from build123d import *

# Parameters (mm, degrees)
SKETCH1_R                = 30
BOSS_EXTRUDE1_DEPTH      = 150
SKETCH3_R                = 57.769734486
BOSS_EXTRUDE2_DEPTH      = 25
BOSS_EXTRUDE2_DEPTH_BACK = 78


with BuildPart() as part:
    # Sketch1 → Boss-Extrude1 (new body)
    with BuildSketch(Plane(origin=(0, 0, 0), x_dir=(1, 0, 0), z_dir=(0, 1, 0))):
        Circle(SKETCH1_R)
    extrude(amount=BOSS_EXTRUDE1_DEPTH)

    # Sketch3 → Boss-Extrude2 (add, two sides)
    with BuildSketch(Plane(origin=(30, 0, 0), x_dir=(0, 0, -1), z_dir=(1, 0, 0))) as boss_extrude2_sk:
        with Locations((22.49423093, 77.731577971)):
            Circle(SKETCH3_R)
    extrude(amount=BOSS_EXTRUDE2_DEPTH)
    extrude(boss_extrude2_sk.sketch, amount=-BOSS_EXTRUDE2_DEPTH_BACK)


solid = part.part
Verification items for the finished model (mm, model axes). A direction names the side the tool comes from. Coordinates: 2 decimals unless noted, no trailing zeros. Order: outer loops, then holes, each group sorted by start corner. A loop starts at its lowest first (then second) coordinate and runs counter-clockwise, first axis right, second up. Notation, with made-up numbers: M 14,26.5 L 36,26.5 A30 ccw 36,57.5 Z; hole C 45,-7 d10. An arc over 180 degrees is marked long. One line per item, written item: value. Start each with the question number.
Item 1: Sectioned sample at B-B (x = 22.5). Enter the section's corners in (y, z).
Item 2: Scan lines: probe 1 along Y at (x, z) = (-24, -23.5); probe 2 along Y at (x, z) = (-43, -52); probe 3 along X at (y, z) = (13, 21.5). Record each from-to range of solid material in increasing order.
Item 3: Sectioned sample at D-D (z = -19). Enter the section's corners in (x, y), then the cut area to 3 significant figures.
Item 4: Sectioned sample at C-C (y = 125). Enter the section's corners in (x, z).
Item 5: Gauge pin test, flat ends, axial feed: pin 1 (1.5 mm diameter, centred on x = -27.5, y = 92, fed in from +Z); pin 2 (1.5 mm diameter, centred on x = -5.5, y = 114.5, fed in from -Z); pin 3 (1 mm diameter, centred on x = 18, z = -39.5, fed in from +Y). Record the tip position at first contact, or that the pin passes through.
Item 6: Sectioned sample at A-A (z = 0). Enter the section's corners in (x, y), then the cut area to 3 significant figures.
Item 7: Access from +Z, -Z, +X, -X, +Y, -Y to the whole of each face (thin tool, end or side, straight path). Record for faces 1 (the cylindrical face through (-6.503, 136.288, 29.287)), 2 (the cylindrical face through (-6.503, 14.517, 29.287)), 3 (the flat face through (0, 0, 0)).
Conclusion:
1. outline: M 0,-19.84 L 20.02,-19.84 A57.77 ccw long 135.44,-19.84 L 150,-19.84 L 150,19.84 L 117.04,19.84 A57.77 ccw 38.43,19.84 L 0,19.84 Z
2. probe 1: y = 19.97 to 135.49
2. probe 2: y = 28.07 to 127.4
2. probe 3: x = -20.92 to 20.92
3. outline: M -48,20.07 L -23.22,20.07 L -23.22,0 L 23.22,0 L 23.22,20.07 L 55,20.07 L 55,135.4 L 23.22,135.4 L 23.22,150 L -23.22,150 L -23.22,135.4 L -48,135.4 Z
3. area: 13,500 mm^2
4. outline: M -48,-55.71 L 55,-55.71 L 55,10.72 L 28.02,10.72 A30 ccw -28.02,10.72 L -48,10.72 Z
5. pin 1: stops at z = 33.67
5. pin 2: stops at z = -67.66
5. pin 3: stops at y = 133.09
6. outline: M -48,24.52 L -30,24.52 L -30,0 L 30,0 L 30,24.52 L 55,24.52 L 55,130.94 L 30,130.94 L 30,150 L -30,150 L -30,130.94 L -48,130.94 Z
6. area: 13,600 mm^2
7. face 1: +Y
7. face 2: -Y
7. face 3: +Z, -Z, +X, -X, -Y
